The listing builds one solid part. Answer for the finished solid, in the listing's coordinates (mm). Face numbers are marked on the shaded views. A direction names the side the tool comes from. Round coordinates to 2 decimals unless told otherwise and drop trailing zeros. Write each loop counter-clockwise with the first axis right and the second up, starting at its lowest first coordinate (ties: lowest second). Pieces come first, ordered by that corner, then holes. Notation, with made-up numbers: (-33, 60) - (6, 60) arc R19 ccw to (6, 78) - close; hole circle Ø1 at (2.5, 54.25). An arc over 180 degrees is marked (long way). Answer as CSV lines item,"result". Start each with the question number.
Item 1: Which of the six approach directions +Z, -Z, +X, -X, +Y, -Y give full straight-line access (tool end or side, diameter ignored) to the marked faces 1 and 2?
Item 2: A cutting plane is placed at B-B on z = 0. Determine the outline of the cut face in (x, y), and give its area (3 significant figures).
Item 3: Straight lines are drawn through the part: line 1 along Z through (x, y) = (0, 24.6); line 2 along X through (y, z) = (24.5, -1.25); line 3 along Z through (x, y) = (-4.5, 21.5). For each, find the intervals that lie inside material, in ascending order. Write a range as [from, to].
Item 4: For a pull along X with two mould halves and no side action, classify the marked faces 3, 4 and 5 as pulls with the +X half, pulls with the -X half, needs draft (parallel to the pull), parting line crosses it, or undercut.
Item 5: A cutting plane is placed at A-A on x = 0. Determine the outline of the cut face in (y, z).
Item 6: A cutting plane is placed at C-C on y = 3.5. Determine the outline of the cut face in (x, z).
Item 7: Flat-ended cylindrical pins translate along their axes: pin 1 (1 mm diameter, centred on x = -3, y = 15.5, fed in from -Z); pin 2 (1 mm diameter, centred on x = 4, y = 11, fed in from -Z); pin 3 (1 mm diameter, centred on x = -5, z = 5.5, fed in from -Y). Find the tip coordinate at first contact, or state that the pin passes through.
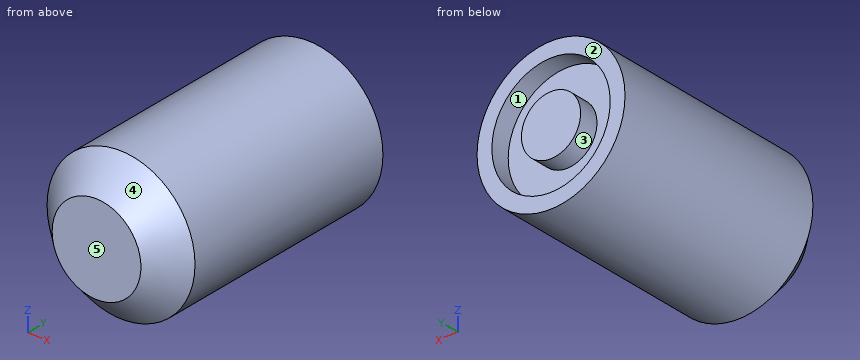
Autodesk Inventor part; units mm, degrees
ref_plane "YZ Plane" through (0, 0, 0) normal (1, 0, 0) x (0, 1, 0)
ref_plane "XZ Plane" through (0, 0, 0) normal (0, 1, 0) x (-1, 0, 0)
ref_plane "XY Plane" through (0, 0, 0) normal (0, 0, 1) x (1, 0, 0)
sketch "Esquisse1" plane through (0, 0, 0) normal (0, 1, 0) x (-1, 0, 0)
  circle A0 centre (0, 0) radius 7.5
  dimension "d0" = 15
extrude "Extrusion1" add sketch "Esquisse1" along normal blind 26
sketch "Esquisse2" plane through (0, 26, 0) normal (0, 1, 0) x (1, 0, 0)
  circle A0 centre (0, 0) radius 6
  circle A1 centre (0, 0) radius 3
  dimension "d3" = 12
  dimension "d4" = 6
extrude "Extrusion2" cut sketch "Esquisse2" against normal blind 2
chamfer "Chanfrein1" distance 3 angle 45 1 edges at (7.5, 0, 0)
properties part number "Pion rond"
Geometry says:
1,face 1,"+Y"
1,face 2,"+Z, -Z, +X, -X, +Y"
2,outline,"(-7.5, 3) - (-4.5, 0) - (4.5, 0) - (7.5, 3) - (7.5, 26) - (6, 26) - (6, 24) - (3, 24) - (3, 26) - (-3, 26) - (-3, 24) - (-6, 24) - (-6, 26) - (-7.5, 26) - close"
2,area,"369 mm^2"
3,line 1,"z = [-7.5, -6], [-3, 3], [6, 7.5]"
3,line 2,"x = [-7.4, -5.87], [-2.73, 2.73], [5.87, 7.4]"
3,line 3,"z = [-6, 6]"
4,face 3,"undercut"
4,face 4,"parting line crosses it"
4,face 5,"needs draft"
5,outline,"(0, -4.5) - (3, -7.5) - (26, -7.5) - (26, -6) - (24, -6) - (24, -3) - (26, -3) - (26, 3) - (24, 3) - (24, 6) - (26, 6) - (26, 7.5) - (3, 7.5) - (0, 4.5) - close"
6,outline,"circle Ø15 at (0, 0)"
7,pin 1,"stops at z = -7.07"
7,pin 2,"stops at z = -6.63"
7,pin 3,"stops at y = 2.43"
